```python
from build123d import *

# Parameters (mm, degrees)
SKETCH1_R           = 42.5
BOSS_EXTRUDE3_DEPTH = 40


with BuildPart() as part:
    # Sketch1 → Boss-Extrude3 (new body)
    with BuildSketch(Plane.XY):
        with BuildLine():
            Line((14.58274905, 79.160170984), (7, 96.492168812))
            Line((7, 96.492168812), (-7, 96.492168812))
            Line((-7, 96.492168812), (-14.58274905, 79.160170984))
            ThreePointArc((-14.58274905, 79.160170984), (-16.735262915, 78.733221802), (-18.875338057, 78.247753024))
            Line((-18.875338057, 78.247753024), (-32.852082622, 90.997139018))
            Line((-32.852082622, 90.997139018), (-45.641719029, 85.302826015))
            Line((-45.641719029, 85.302826015), (-45.519346366, 66.385076234))
            ThreePointArc((-45.519346366, 66.385076234), (-47.312109753, 65.119532483), (-49.069707737, 63.805587708))
            Line((-49.069707737, 63.805587708), (-67.023741707, 69.767877205))
            Line((-67.023741707, 69.767877205), (-76.391570197, 59.363849648))
            Line((-76.391570197, 59.363849648), (-68.585235165, 42.131398713))
            ThreePointArc((-68.585235165, 42.131398713), (-69.708262997, 40.246084406), (-70.779479165, 38.330856621))
            Line((-70.779479165, 38.330856621), (-89.60638696, 36.475115601))
            Line((-89.60638696, 36.475115601), (-93.932624881, 23.160324373))
            Line((-93.932624881, 23.160324373), (-79.792113727, 10.592819603))
            ThreePointArc((-79.792113727, 10.592819603), (-80.05122429, 8.413722711), (-80.250835633, 6.2283722))
            Line((-80.250835633, 6.2283722), (-96.695273858, -3.124524856))
            Line((-96.695273858, -3.124524856), (-95.231875373, -17.047831391))
            Line((-95.231875373, -17.047831391), (-77.202210937, -22.77735425))
            ThreePointArc((-77.202210937, -22.77735425), (-76.55260166, -24.873448077), (-75.846093565, -26.951054358))
            Line((-75.846093565, -26.951054358), (-87.064669458, -42.18390658))
            Line((-87.064669458, -42.18390658), (-80.064669458, -54.308262233))
            Line((-80.064669458, -54.308262233), (-61.263344515, -52.209116626))
            ThreePointArc((-61.263344515, -52.209116626), (-59.817338744, -53.859773725), (-58.32687288, -55.470398775))
            Line((-58.32687288, -55.470398775), (-62.37979275, -73.949307627))
            Line((-62.37979275, -73.949307627), (-51.053554829, -82.178301159))
            Line((-51.053554829, -82.178301159), (-34.731489268, -72.613448433))
            ThreePointArc((-34.731489268, -72.613448433), (-32.739114537, -73.533255194), (-30.72240599, -74.39840731))
            Line((-30.72240599, -74.39840731), (-26.908883174, -92.928201578))
            Line((-26.908883174, -92.928201578), (-13.214816763, -95.838965249))
            Line((-13.214816763, -95.838965249), (-2.194244, -80.462255334))
            ThreePointArc((-2.194244, -80.462255334), (0, -80.492168812), (2.194244, -80.462255334))
            Line((2.194244, -80.462255334), (13.214816763, -95.838965249))
            Line((13.214816763, -95.838965249), (26.908883174, -92.928201578))
            Line((26.908883174, -92.928201578), (30.72240599, -74.39840731))
            ThreePointArc((30.72240599, -74.39840731), (32.739114537, -73.533255194), (34.731489268, -72.613448433))
            Line((34.731489268, -72.613448433), (51.053554829, -82.178301159))
            Line((51.053554829, -82.178301159), (62.37979275, -73.949307627))
            Line((62.37979275, -73.949307627), (58.32687288, -55.470398775))
            ThreePointArc((58.32687288, -55.470398775), (59.817338744, -53.859773725), (61.263344515, -52.209116626))
            Line((61.263344515, -52.209116626), (80.064669458, -54.308262233))
            Line((80.064669458, -54.308262233), (87.064669458, -42.18390658))
            Line((87.064669458, -42.18390658), (75.846093565, -26.951054358))
            ThreePointArc((75.846093565, -26.951054358), (76.55260166, -24.873448077), (77.202210937, -22.77735425))
            Line((77.202210937, -22.77735425), (95.231875373, -17.047831391))
            Line((95.231875373, -17.047831391), (96.695273858, -3.124524856))
            Line((96.695273858, -3.124524856), (80.250835633, 6.2283722))
            ThreePointArc((80.250835633, 6.2283722), (80.05122429, 8.413722711), (79.792113727, 10.592819603))
            Line((79.792113727, 10.592819603), (93.932624881, 23.160324373))
            Line((93.932624881, 23.160324373), (89.60638696, 36.475115601))
            Line((89.60638696, 36.475115601), (70.779479165, 38.330856621))
            ThreePointArc((70.779479165, 38.330856621), (69.708262997, 40.246084406), (68.585235165, 42.131398713))
            Line((68.585235165, 42.131398713), (76.391570197, 59.363849648))
            Line((76.391570197, 59.363849648), (67.023741707, 69.767877205))
            Line((67.023741707, 69.767877205), (49.069707737, 63.805587708))
            ThreePointArc((49.069707737, 63.805587708), (47.312109753, 65.119532483), (45.519346366, 66.385076234))
            Line((45.519346366, 66.385076234), (45.641719029, 85.302826015))
            Line((45.641719029, 85.302826015), (32.852082622, 90.997139018))
            Line((32.852082622, 90.997139018), (18.875338057, 78.247753024))
            ThreePointArc((18.875338057, 78.247753024), (16.735262915, 78.733221802), (14.58274905, 79.160170984))
        make_face()
        Circle(SKETCH1_R, mode=Mode.SUBTRACT)
    extrude(amount=BOSS_EXTRUDE3_DEPTH)


solid = part.part
```
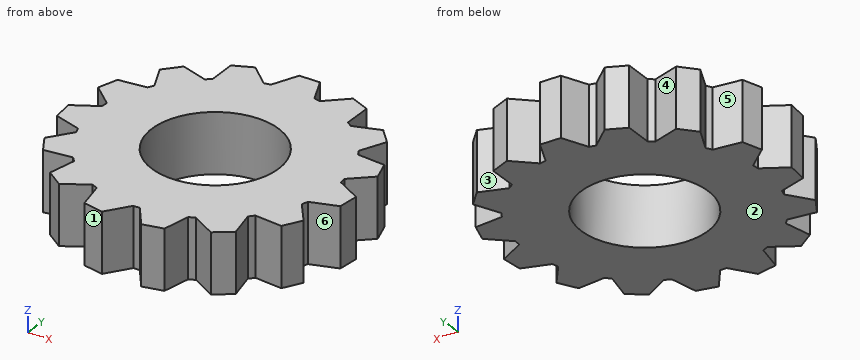
Geometry check sheet. Reference: the model listing, model coordinates, mm. Face numbers are marked on the shaded views. A direction names the side the tool comes from. Coordinates: 2 decimals unless noted, no trailing zeros. Order: outer loops, then holes, each group sorted by start corner. A loop starts at its lowest first (then second) coordinate and runs counter-clockwise, first axis right, second up. Notation, with made-up numbers: (-15.75, -7) - (-10.75, -7) arc R17 cw to (-10.75, 4) - close; hole circle Ø10 at (-39.5, 30). An arc over 180 degrees is marked (long way). Answer in a Markdown table with one row per item. Add a question column.
1. Draft check along X on the marked faces 1, 2 and 3. Enter one of: +X half, -X half, draft (parallel to the pull), parting line (faces both ways), or undercut.
2. Section check A-A (x = 84). Enter the section's corners in (y, z), plus the area to 3 significant figures.
3. Gauge pin test, flat ends, axial feed: pin 1 Ø3 at (x, z) = (42, 4.5) entering from -Y; pin 2 Ø1.5 at (x, z) = (43.5, 5) entering from -Y; pin 3 Ø3 at (y, z) = (25.5, 26.5) entering from +X. Record the tip position at first contact, or that the pin passes through.
4. Access from +Z, -Z, +X, -X, +Y, -Y to the whole of each face (thin tool, end or side, straight path). Record for the marked faces 4, 5 and 6.
5. Material ranges on L1, parallel to Y at x = 0, z = 18; L2, parallel to Y at x = -33.5, z = 29; L3, parallel to X at y = -31.5, z = 15.5, recorded low to high. Write a range as [from, to].
6. Section check B-B (y = 2.5). Enter the section's corners in (x, z).
Data:
| question | item | result |
|---|---|---|
| 1 | face 1 | -X half |
| 1 | face 2 | draft |
| 1 | face 3 | undercut |
| 2 | outline | (-47.49, 0) - (-38.02, 0) - (-38.02, 40) - (-47.49, 40) - close; (-20.62, 0) - (4.1, 0) - (4.1, 40) - (-20.62, 40) - close; (14.33, 0) - (37.03, 0) - (37.03, 40) - (14.33, 40) - close |
| 2 | area | 2,280 mm² |
| 3 | pin 1 | stops at y = -77.75 |
| 3 | pin 2 | stops at y = -78.19 |
| 3 | pin 3 | stops at x = 93.66 |
| 4 | face 4 | +Z, -Z, +Y |
| 4 | face 5 | +Z, -Z, -X |
| 4 | face 6 | +Z, -Z, +X |
| 5 | L1 | y = [-80.49, -42.5], [42.5, 96.49] |
| 5 | L2 | y = [-73.19, -26.15], [26.15, 90.71] |
| 5 | L3 | x = [-79.2, -28.53], [28.53, 79.2] |
| 6 | outline | (-86.81, 0) - (-42.43, 0) - (-42.43, 40) - (-86.81, 40) - close; (42.43, 0) - (86.81, 0) - (86.81, 40) - (42.43, 40) - close |
